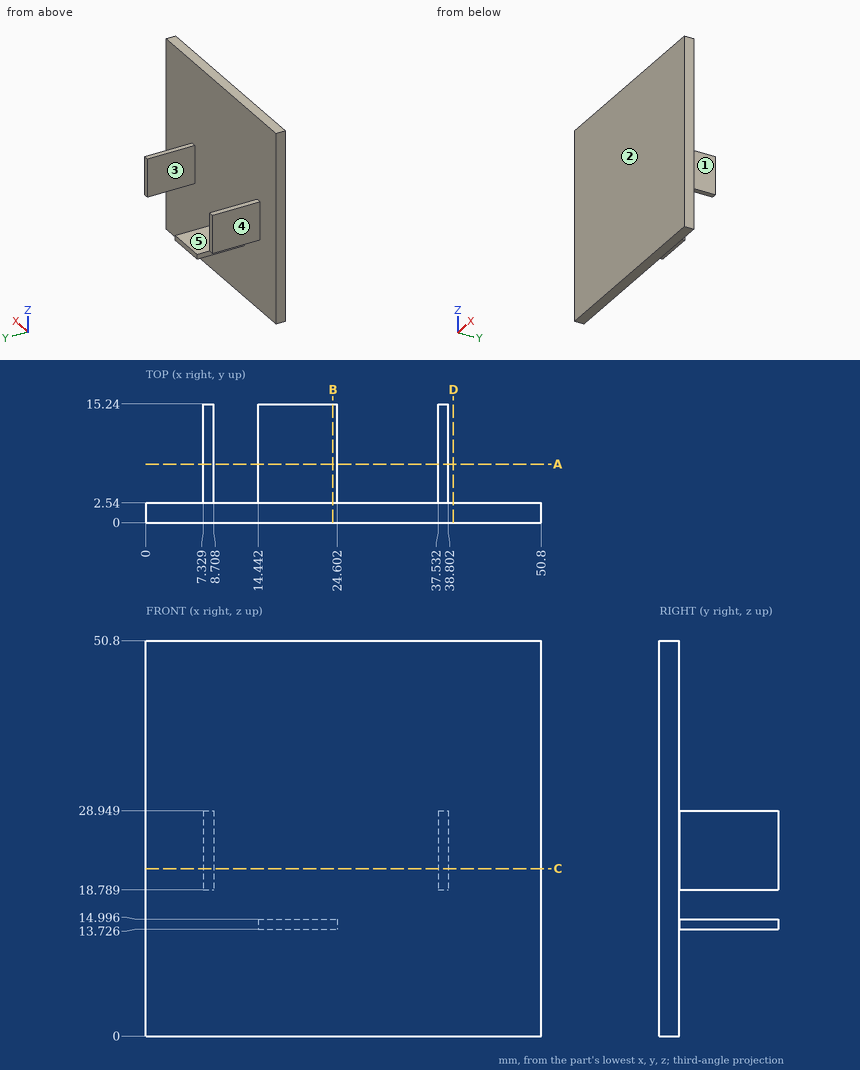
Geometry check sheet. Reference: drawing and pictorial views, mm from the part's lowest x, y, z. A direction names the side the tool comes from. Round coordinates to 2 decimals unless told otherwise and drop trailing zeros. Write each loop counter-clockwise with the first axis right and the second up, starting at its lowest first coordinate (ties: lowest second). Pieces come first, ordered by that corner, then holes. Notation, with made-up numbers: (12.25, -15.5) -> (46.25, -15.5) arc R27 ccw to (46.25, 12.5) -> close; hole circle Ø1 at (71.5, 10). An arc over 180 degrees is marked (long way). Put each result on its own line as item: value.
1) Release check for a two-part mould opening along X. For the marked faces 1, 2 and 3 record: pulls with the +X half, pulls with the -X half, needs draft (parallel to the pull), parting line crosses it, or undercut.
Recorded:
face 1: pulls with the +X half
face 2: needs draft
face 3: undercut
2) Cross-section at A-A, the plane y = 7.5. Enter the section's corners in (x, z) (1 decimal).
Recorded:
outline: (7.3, 18.8) -> (8.7, 18.8) -> (8.7, 28.9) -> (7.3, 28.9) -> close; (14.4, 13.7) -> (24.6, 13.7) -> (24.6, 15) -> (14.4, 15) -> close; (37.5, 18.8) -> (38.8, 18.8) -> (38.8, 28.9) -> (37.5, 28.9) -> close
3) Access from +Z, -Z, +X, -X, +Y, -Y to the whole of each face (thin tool, end or side, straight path). Record for the marked faces 4 and 5.
Recorded:
face 4: +Z, -Z, -X, +Y
face 5: +Z, +X, -X, +Y
4) Cross-section at C-C, the plane z = 21.5. Enter the section's corners in (x, y), plus the area to 3 significant figures.
Recorded:
outline: (0, 0) -> (50.8, 0) -> (50.8, 2.54) -> (38.8, 2.54) -> (38.8, 15.24) -> (37.53, 15.24) -> (37.53, 2.54) -> (8.71, 2.54) -> (8.71, 15.24) -> (7.33, 15.24) -> (7.33, 2.54) -> (0, 2.54) -> close
area: 163 mm2
5) Thickness scan on probe 1 along X at (y, z) = (3.25, 27.5); probe 2 along Y at (x, z) = (46, 43.5); probe 3 along Z at (x, y) = (22, 7.75) (1 decimal). Record the ranges inside material, lowest first. Write a range as from..to.
Recorded:
probe 1: x = 7.33..8.71, 37.53..38.8
probe 2: y = 0..2.54
probe 3: z = 13.7..15
6) Depth check by flat-ended pin: P1, Ø5, axis at y = 6, z = 25.5, coming from the -X side; P2, Ø3, axis at x = 41.5, y = 6, coming from the -Z side; P3, Ø1.4, axis at y = 10.5, z = 14.5, coming from the +X side; P4, Ø3, axis at y = 11.5, z = 24.5, coming from the +X side. Enter the tip coordinate at first touch or a pass-through.
Recorded:
P1: stops at x = 7.33
P2: passes through
P3: stops at x = 24.6
P4: stops at x = 38.8
7) Cross-section at B-B, the plane x = 24. Enter the section's corners in (y, z) (1 decimal).
Recorded:
outline: (0, 0) -> (2.5, 0) -> (2.5, 13.7) -> (15.2, 13.7) -> (15.2, 15) -> (2.5, 15) -> (2.5, 50.8) -> (0, 50.8) -> close
8) Cross-section at D-D, the plane x = 39.5. Enter the section's corners in (y, z).
Recorded:
outline: (0, 0) -> (2.54, 0) -> (2.54, 50.8) -> (0, 50.8) -> close
